Autodesk Fusion 360 part; units mm, degrees
sketch "Sketch1" plane through (0, 0, 0) normal (0, 0, 1) x (1, 0, 0)
  line L0 (0, 0) -> (66, 0) construction
  line L1 (66, 0) -> (66, -42) construction
  line L2 (66, -42) -> (0, -42) construction
  line L3 (0, -42) -> (0, 0)
  line L4 (66, 0) -> (54, 0) construction
  line L5 (54, 0) -> (54, -12) construction
  line L6 (54, -12) -> (66, -12) construction
  line L7 (66, -12) -> (66, 0) construction
  line L8 (66, -42) -> (54, -42) construction
  line L9 (54, -42) -> (54, -30) construction
  line L10 (54, -30) -> (66, -30) construction
  line L11 (66, -30) -> (66, -42) construction
  line L12 (54, 0) -> (66, -12)
  line L13 (66, -30) -> (54, -42)
  line L14 (0, -42) -> (54, -42)
  line L15 (0, 0) -> (54, 0)
  line L16 (66, -12) -> (66, -30)
  line L17 (0, 0) -> (12, 0)
  line L18 (12, 0) -> (12, -42)
  line L19 (12, -42) -> (0, -42)
  line L20 (0, -42) -> (0, 0)
  line L21 (66, -21) -> (12, -21)
  line L22 (12, -21) -> (12, -15)
  line L23 (12, -21) -> (12, -27)
  line L24 (12, -27) -> (66, -27)
  line L25 (12, -15) -> (66, -15)
  dimension "d1" = 66
  dimension "d2" = 42
  dimension "d3" = 12
  dimension "d4" = 12
  dimension "d5" = 12
  dimension "d6" = 12
  dimension "d7" = 42
  dimension "d8" = 12
  dimension "d9" = 6
  dimension "d10" = 6
extrude "Extrude1" add sketch "Sketch1" along normal blind 60 contours L3 L14 L15 L17 L18 L19 L20 L22 L23 makes body 1
extrude "Extrude2" add sketch "Sketch1" along normal blind 12 contours L13 L14 L16 L18 L24 | L12 L15 L16 L18 L25 | L16 L18 L21 L23 L24 | L16 L18 L21 L22 L25 bodies 1
sketch "Sketch2" plane through (0, 0, 0) normal (-1, 0, 0) x (0, -1, 0)
  line L0 (0, 0) -> (42, 0)
  line L1 (42, 0) -> (42, 60)
  line L2 (42, 60) -> (0, 60)
  line L3 (0, 60) -> (0, 0)
  line L4 (0, 60) -> (42, 60)
  line L5 (42, 60) -> (42, 0)
  line L6 (42, 0) -> (0, 0)
  line L7 (0, 0) -> (0, 60)
  circle A0 centre (21, 39) radius 21
  dimension "d15" = 42
extrude "Extrude3" cut sketch "Sketch2" against normal blind 15 contours L2 L3 L4 L7 A0 | L1 L2 L4 L5 A0 bodies 1
extrude "Extrude4" add sketch "Sketch1" along normal blind 54 separate body contours L16 L18 L21 L23 L24 | L16 L18 L21 L22 L25 makes body 2
sketch "Sketch3" plane through (0, -15, 0) normal (0, 1, 0) x (-1, 0, 0)
  line L0 (-66, 0) -> (-12, 0)
  line L1 (-12, 0) -> (-12, 54)
  line L2 (-12, 54) -> (-66, 54)
  line L3 (-66, 54) -> (-66, 0)
  line L4 (-66, 11.9878) -> (-12, 54)
extrude "Extrude5" cut sketch "Sketch3" against normal blind 25 contours L2 L3 L4 bodies 1 2
combine "Combine1" operation add target body 1 tool bodies 2
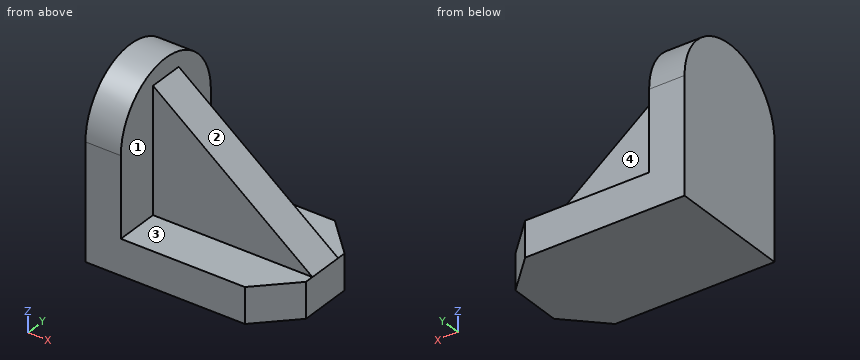
Geometry: final body of the model. Coordinates: model frame, mm. Face numbers are marked on the shaded views. A direction names the side the tool comes from. Give positions to 0.01 mm unless a question says otherwise; leave off trailing zeros. Write each loop counter-clockwise with the first axis right and the second up, starting at its lowest first coordinate (ties: lowest second). Pieces come first, ordered by that corner, then holes. Notation, with made-up numbers: (44.25, 83.5) -> (62.25, 83.5) arc R23 ccw to (62.25, 101.5) -> close; hole circle Ø11 at (40.5, 10.5). An arc over 180 degrees is marked (long way). Answer in a Markdown table with one row per item.
(1) Set-up query: the marked faces 1, 2, 3 and 4. Return all of +Z, -Z, +X, -X, +Y, -Y with unobstructed straight access to the full face (end or side cutting, diameter ignored); none if empty.
Answers below:
| item | result |
|---|---|
| face 1 | +Z, +X |
| face 2 | +Z, +X, +Y, -Y |
| face 3 | +Z, +X, -Y |
| face 4 | +Z, +X, +Y |
(2) Section query B-B on x = 49. Return loops of the section in (y, z).
Answers below:
| item | result |
|---|---|
| outline | (-42, 0) -> (0, 0) -> (0, 12) -> (-15, 12) -> (-15, 25.21) -> (-27, 25.21) -> (-27, 12) -> (-42, 12) -> close |
(3) Pin query (flat end, axial travel): pin 1 (21 mm diameter, centred on x = 26.5, z = 33, fed in from -Y); pin 2 (2 mm diameter, centred on x = 25, z = 37.5, fed in from +Y); pin 3 (1 mm diameter, centred on y = -31, z = 17, fed in from +X). Return the tip coordinate at first contact, or that it passes through.
Answers below:
| item | result |
|---|---|
| pin 1 | y = -27 |
| pin 2 | y = -15 |
| pin 3 | x = 12 |
(4) Ray query, line 1 along Z through (x, y) = (47.5, -3.5); line 2 along Y through (x, z) = (22, 27). Return the intervals inside material, ascending. Write a range as [from, to].
Answers below:
| item | result |
|---|---|
| line 1 | [0, 12] |
| line 2 | [-27, -15] |
(5) Section query A-A on z = 49. Return loops of the section in (x, y), then the cut area to 3 significant figures.
Answers below:
| item | result |
|---|---|
| outline | (0, -39.47) -> (12, -39.47) -> (12, -27) -> (18.43, -27) -> (18.43, -15) -> (12, -15) -> (12, -2.53) -> (0, -2.53) -> close |
| area | 520 mm^2 |
(6) Section query D-D on x = 5.5. Return loops of the section in (y, z).
Answers below:
| item | result |
|---|---|
| outline | (-42, 0) -> (0, 0) -> (0, 39) arc R21 ccw to (-42, 39) -> close |
(7) Section query C-C on y = -21. Return loops of the section in (x, z), then the cut area to 3 significant figures.
Answers below:
| item | result |
|---|---|
| outline | (0, 0) -> (66, 0) -> (66, 11.99) -> (12, 54) -> (12, 60) -> (0, 60) -> close |
| area | 2,500 mm^2 |
